from build123d import *

# Parameters (mm, degrees)
CUT_EXTRUDE1_DEPTH     = 5
CUT_EXTRUDE3_DEPTH     = 45
SKETCH8_R              = 40
CUT_EXTRUDE4_DEPTH     = 32
FILLET1_R              = 7
FILLET2_R              = 8
CUT_REVOLVE1_START     = 17
CUT_REVOLVE1_DEPTH     = 30.5
SKETCH18_W             = 13
SKETCH18_H             = 8
CUT_EXTRUDE13_DEPTH    = 5
SKETCH20_W             = 84
SKETCH20_H             = 7
CUT_EXTRUDE15_DEPTH    = 5
SKETCH19_R             = 1.5
CUT_EXTRUDE14_DEPTH    = 12
FILLET3_R              = 4
SKETCH21_W             = 16
SKETCH21_H             = 5
CUT_EXTRUDE16_DEPTH    = 5
CIRPATTERN1_COUNT      = 4
SKETCH22_W             = 5
SKETCH22_H             = 12
BOSS_EXTRUDE1_DEPTH    = 1.5
SKETCH23_W             = 5
SKETCH23_H             = 4.4
SKETCH23_H_2           = 4
BOSS_EXTRUDE2_DEPTH    = 17
SKETCH24_W             = 2
SKETCH24_H             = 3
BOSS_EXTRUDE3_DEPTH    = 2
CIRPATTERN2_COUNT      = 5
INTERSECT1_START       = 47.5
INTERSECT1_OUTLINE_R   = 42
INTERSECT1_OUTLINE_W   = 13
INTERSECT1_OUTLINE_H   = 8
INTERSECT1_DEPTH       = 7.5
INTERSECT2_OUTLINE_W   = 86
INTERSECT2_OUTLINE_H   = 86
INTERSECT2_OUTLINE_W_2 = 5
INTERSECT2_OUTLINE_H_2 = 16
INTERSECT2_OUTLINE_W_3 = 16
INTERSECT2_OUTLINE_H_3 = 5
INTERSECT2_DEPTH       = 14
SKETCH28_W             = 10
SKETCH28_H             = 10
BOSS_EXTRUDE4_DEPTH    = 2.5
BOSS_EXTRUDE4_DRAFT    = -41


# Read off the part's stored shape, not the designer's step: Cut-Revolve1, Intersect1, Intersect2
with BuildPart() as part:
    # Sketch1 → Revolve1 (revolve)
    with BuildSketch(Plane.XY, mode=Mode.PRIVATE) as revolve1_sk:
        with BuildLine():
            Line((37, 55), (0, 55))
            Line((0, 55), (0, 11.5))
            Line((0, 11.5), (22.5, 11.5))
            Line((22.5, 11.5), (22.5, 0))
            Line((22.5, 0), (25, 0))
            Line((25, 0), (25, 11.5))
            Line((25, 11.5), (42, 11.5))
            Line((42, 11.5), (42, 50))
            ThreePointArc((42, 50), (40.535533906, 53.535533906), (37, 55))
        make_face()
    revolve(revolve1_sk.sketch.rotate(Axis((0, 2, 0), (0, 1, 0)), 90), axis=Axis((0, 2, 0), (0, 1, 0)))

    # Sketch5 → Cut-Extrude1 (cut)
    with BuildSketch(Plane(origin=(0, 55, 0), x_dir=(1, 0, 0), z_dir=(0, 1, 0))):
        with BuildLine():
            Line((-42, 0), (-40, 0))
            Line((-40, 0), (40, 0))
            Line((40, 0), (42, 0))
            ThreePointArc((42, 0), (0, 42), (-42, 0))
        make_face()
    extrude(amount=-CUT_EXTRUDE1_DEPTH, mode=Mode.SUBTRACT)

    # Sketch7 → Cut-Extrude3 (cut)
    with BuildSketch(Plane.XZ.offset(-11.5)):
        with BuildLine():
            Line((-21, 0), (21, 0))
            ThreePointArc((21, 0), (0, -21), (-21, 0))
        make_face()
    extrude(amount=-CUT_EXTRUDE3_DEPTH, mode=Mode.SUBTRACT)

    # Sketch8 → Cut-Extrude4 (cut)
    with BuildSketch(Plane(origin=(0, 47.5, 0), x_dir=(1, 0, 0), z_dir=(0, 1, 0))):
        with Locations(Location((0, 0, 0), (0, 0, 270))):
            Circle(SKETCH8_R)
        with BuildLine():
            Line((22.912878475, -2), (-22.912878475, -2))
            ThreePointArc((-22.912878475, -2), (0, 23), (22.912878475, -2))
        make_face(mode=Mode.SUBTRACT)
    extrude(amount=-CUT_EXTRUDE4_DEPTH, mode=Mode.SUBTRACT)

    # Fillet1
    fillet1_edges = [part.edges().sort_by_distance(p)[0] for p in [
        (21, 30.75, 0),
        (-21, 30.75, 0),
    ]]
    fillet(fillet1_edges, radius=FILLET1_R)

    # Fillet2
    fillet2_edges = [part.edges().sort_by_distance(p)[0] for p in [
        (-22.912878475, 31.5, 2),
        (22.912878475, 31.5, 2),
    ]]
    fillet(fillet2_edges, radius=FILLET2_R)

    # Cut-Revolve1 outline → Cut-Revolve1 (cut)
    with BuildSketch(Plane(origin=(0, 0, 0), x_dir=(1, 0, 0), z_dir=(0, 1, 0)).offset(CUT_REVOLVE1_START)):
        with BuildLine():
            Line((-34.641016151, -20), (-36.373066959, -21))
            ThreePointArc((-36.373066959, -21), (0, -42), (36.373066959, -21))
            Line((36.373066959, -21), (34.641016151, -20))
            ThreePointArc((34.641016151, -20), (0, -40), (-34.641016151, -20))
        make_face()
    extrude(amount=CUT_REVOLVE1_DEPTH, mode=Mode.SUBTRACT)

    # Sketch18 → Cut-Extrude13 (cut)
    with BuildSketch(Plane(origin=(0, 50, 0), x_dir=(1, 0, 0), z_dir=(0, 1, 0))):
        with Locations((0.796512215, 32.951769165)):
            Rectangle(SKETCH18_W, SKETCH18_H)
    extrude(amount=-CUT_EXTRUDE13_DEPTH, mode=Mode.SUBTRACT)

    # Sketch20 → Cut-Extrude15 (cut)
    with BuildSketch(Plane(origin=(0, 55, 0), x_dir=(1, 0, 0), z_dir=(0, 1, 0))):
        with Locations((0, -3.5)):
            Rectangle(SKETCH20_W, SKETCH20_H)
    extrude(amount=-CUT_EXTRUDE15_DEPTH, mode=Mode.SUBTRACT)

    # Sketch19 → Cut-Extrude14 (cut)
    with BuildSketch(Plane(origin=(0, 0, 7), x_dir=(-1, 0, 0), z_dir=(0, 0, -1))):
        with Locations((0, 52.5)):
            Circle(SKETCH19_R)
        with Locations((-29.412558482, 52.5)):
            Circle(SKETCH19_R)
        with Locations((29.412558482, 52.5)):
            Circle(SKETCH19_R)
    extrude(amount=-CUT_EXTRUDE14_DEPTH, mode=Mode.SUBTRACT)

    # Fillet3
    fillet3_edges = [part.edges().sort_by_distance(p)[0] for p in [
        (0, 11.5, 42),
    ]]
    fillet(fillet3_edges, radius=FILLET3_R)

    # Sketch21 → Cut-Extrude16 (cut)
    with BuildSketch(Plane(origin=(0, 15.5, 0), x_dir=(1, 0, 0), z_dir=(0, 1, 0))):
        with Locations((0, -29.5)):
            Rectangle(SKETCH21_W, SKETCH21_H)
    cut_extrude16 = extrude(amount=-CUT_EXTRUDE16_DEPTH, mode=Mode.SUBTRACT)

    # CirPattern1: Cut-Extrude16 ×4 about axis
    cirpattern1_axis = Axis((0, 0, 0), (0, 1, 0))
    for i in range(1, CIRPATTERN1_COUNT):
        add(cut_extrude16.rotate(cirpattern1_axis, i * 360 / CIRPATTERN1_COUNT), mode=Mode.SUBTRACT)

    # Sketch22 → Boss-Extrude1 (add)
    with BuildSketch(Plane(origin=(0, 15.5, 0), x_dir=(1, 0, 0), z_dir=(0, 1, 0))):
        with Locations((35.5, -4)):
            Rectangle(SKETCH22_W, SKETCH22_H)
    extrude(amount=BOSS_EXTRUDE1_DEPTH)

    # Sketch23 → Boss-Extrude2 (add)
    with BuildSketch(Plane(origin=(0, 17, 0), x_dir=(1, 0, 0), z_dir=(0, 1, 0))):
        with Locations((35.5, -0.2)):
            Rectangle(SKETCH23_W, SKETCH23_H)
        with Locations((35.5, -8)):
            Rectangle(SKETCH23_W, SKETCH23_H_2)
    extrude(amount=BOSS_EXTRUDE2_DEPTH)

    # Sketch24 → Boss-Extrude3 (add)
    with BuildSketch(Plane.XZ):
        with Locations((0, -22.5)):
            Rectangle(SKETCH24_W, SKETCH24_H)
    boss_extrude3 = extrude(amount=-BOSS_EXTRUDE3_DEPTH)

    # CirPattern2: Boss-Extrude3 ×5 about axis
    cirpattern2_axis = Axis((0, 0, 0), (0, 1, 0))
    for i in range(1, CIRPATTERN2_COUNT):
        add(boss_extrude3.rotate(cirpattern2_axis, i * 360 / CIRPATTERN2_COUNT))

    # Intersect1 outline → Intersect1 (cut)
    with BuildSketch(Plane(origin=(0, 0, 0), x_dir=(1, 0, 0), z_dir=(0, 1, 0)).offset(INTERSECT1_START)):
        Circle(INTERSECT1_OUTLINE_R)
        with BuildLine():
            Line((12.124355653, 0), (-12.124355653, 0))
            ThreePointArc((-12.124355653, 0), (-18.186533479, 3.5), (-18.186533479, 10.5))
            ThreePointArc((-18.186533479, 10.5), (0, 21), (18.186533479, 10.5))
            ThreePointArc((18.186533479, 10.5), (18.186533479, 3.5), (12.124355653, 0))
        make_face(mode=Mode.SUBTRACT)
        with Locations((0.796512215, 32.951769165)):
            Rectangle(INTERSECT1_OUTLINE_W, INTERSECT1_OUTLINE_H, mode=Mode.SUBTRACT)
    extrude(amount=INTERSECT1_DEPTH, mode=Mode.SUBTRACT)

    # Intersect2 outline → Intersect2 (cut)
    with BuildSketch(Plane(origin=(0, 0, 0), x_dir=(1, 0, 0), z_dir=(0, 1, 0))):
        Rectangle(INTERSECT2_OUTLINE_W, INTERSECT2_OUTLINE_H)
        with Locations((29.5, 0)):
            Rectangle(INTERSECT2_OUTLINE_W_2, INTERSECT2_OUTLINE_H_2, mode=Mode.SUBTRACT)
        with Locations((0, -29.5)):
            Rectangle(INTERSECT2_OUTLINE_W_3, INTERSECT2_OUTLINE_H_3, mode=Mode.SUBTRACT)
        with Locations((0, 29.5)):
            Rectangle(INTERSECT2_OUTLINE_W_3, INTERSECT2_OUTLINE_H_3, mode=Mode.SUBTRACT)
        with Locations((-29.5, 0)):
            Rectangle(INTERSECT2_OUTLINE_W_2, INTERSECT2_OUTLINE_H_2, mode=Mode.SUBTRACT)
    extrude(amount=INTERSECT2_DEPTH, mode=Mode.SUBTRACT)


with BuildPart() as boss_extrude4_tool:
    # Sketch28 → Boss-Extrude4 (with draft: the straight prism first)
    with BuildSketch(Plane(origin=(21.747727085, 0, 0), x_dir=(0, 0, -1), z_dir=(1, 0, 0))):
        with Locations((3.079158512, 35.232399588)):
            Rectangle(SKETCH28_W, SKETCH28_H)
    extrude(amount=-BOSS_EXTRUDE4_DEPTH)
    # Boss-Extrude4: the draft: its side faces are tilted about the plane it starts from
    boss_extrude4_sides = [boss_extrude4_tool.faces().sort_by_distance(p)[0] for p in [
        (20.497727085, 35.232399588, 1.920841488),
        (20.497727085, 30.232399588, -3.079158512),
        (20.497727085, 35.232399588, -8.079158512),
        (20.497727085, 40.232399588, -3.079158512),
    ]]
    draft(boss_extrude4_sides, Plane(origin=(21.747727085, 0, 0), x_dir=(0, 0, -1), z_dir=(1, 0, 0)), BOSS_EXTRUDE4_DRAFT)


with BuildPart() as part_1:
    add(part.part)

    # Boss-Extrude4: add boss_extrude4_tool
    add(boss_extrude4_tool.part)


solid = part_1.part
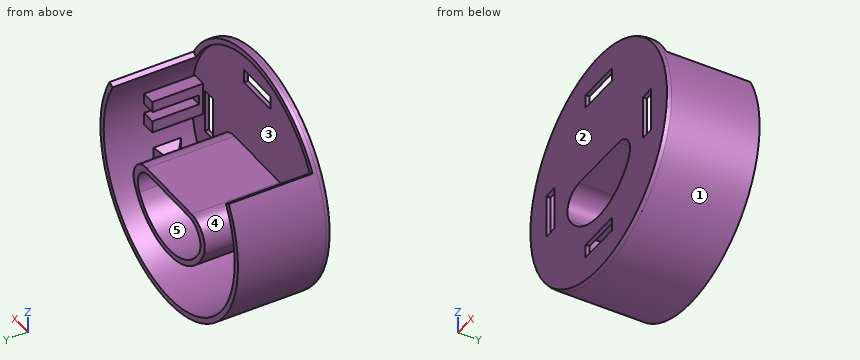
Design review of the part built by this model. Coordinates are the model's own, in mm. Face numbers are marked on the shaded views. A direction names the side the tool comes from. Coordinates: 2 decimals unless noted, no trailing zeros. Order: outer loops, then holes, each group sorted by start corner. A loop starts at its lowest first (then second) coordinate and runs counter-clockwise, first axis right, second up. Notation, with made-up numbers: (77, 11.25) -> (113, 11.25) arc R31 cw to (113, 47.25) -> close; hole circle Ø10 at (45.5, -35). An arc over 180 degrees is marked (long way). Use one line per item in the form item = value. Start each with the question number.
(1) The part is to be moulded in two halves that separate along X. For the marked faces 1, 2 and 3, say which applies: +X half, -X half, draft (parallel to the pull), parting line (faces both ways), or undercut.
(2) Add section A-A on y = 43. State the section outline as (x, z) points, plus the area to 3 significant figures.
(3) Add section B-B on x = 0. State the section outline as (y, z) points.
(4) For the marked faces 4 and 5, list the 3-axis set-ups (+Z, -Z, +X, -X, +Y, -Y) from which the entire face can be reached by the end or side of a thin tool; tool diameter is ignored.
(5) For probe 1 along Z at (x, y) = (-8.5, 44); probe 2 along Z at (x, y) = (-19.5, 38.5); probe 3 along Y at (x, z) = (-13, -21), list the stretches that pass through material, from the lowest coordinate up.
(6) Insertion check: pin 1 (1.2 mm diameter, centred on x = -2.5, y = 15, fed in from -Z); pin 2 (8 mm diameter, centred on x = 21.5, z = -19, fed in from +Y); pin 3 (1.6 mm diameter, centred on y = 14.5, z = -3.5, fed in from +X). Each pin has a flat end and moves straight along its axis. Give the tip position at first contact, or say it passes through.
Answer block:
q1.face_1 = parting line
q1.face_2 = draft
q1.face_3 = undercut
q2.outline = (-36.37, 21) arc R42 ccw (long way) to (36.37, 21) -> (34.64, 20) arc R40 cw (long way) to (-34.64, 20) -> close; (-21.08, -9.2) arc R23 ccw to (21.08, -9.2) arc R8 ccw to (13.75, 2) -> (-13.75, 2) arc R8 ccw to start; hole (-18.19, -10.5) arc R21 ccw to (18.19, -10.5) arc R7 ccw to (12.12, 0) -> (-12.12, 0) arc R7 ccw to start
q2.area = 572 mm²
q3.outline = (14, -41.71) arc R4 ccw to (15.5, -42) -> (47.5, -42) -> (47.5, -40) -> (15.5, -40) -> (15.5, -32) -> (14, -32) -> close; (14, -27) -> (15.5, -27) -> (15.5, -23) -> (47.5, -23) -> (47.5, -21) -> (14, -21) -> close; (14, 0) -> (47.5, 0) -> (47.5, 2) -> (15.5, 2) -> (15.5, 27) -> (14, 27) -> close; (14, 32) -> (15.5, 32) -> (15.5, 40) -> (17, 40) -> (17, 42) -> (15.5, 42) arc R4 ccw to (14, 41.71) -> close
q4.face_4 = +Y
q4.face_5 = +Y, -Y
q5.probe_1 = -41.13 to -39.09, -21.37 to -19.2, 0 to 2
q5.probe_2 = -37.2 to -34.92, -12.2 to -0.44
q5.probe_3 = 14 to 15.5
q6.pin_1 = -41.95
q6.pin_2 = 15.5
q6.pin_3 = 41.88
